Autodesk Inventor part; units mm, degrees
ref_plane "YZ Plane" through (0, 0, 0) normal (1, 0, 0) x (0, 1, 0)
ref_plane "XZ Plane" through (0, 0, 0) normal (0, 1, 0) x (-1, 0, 0)
ref_plane "XY Plane" through (0, 0, 0) normal (0, 0, 1) x (1, 0, 0)
sketch "Sketch1" plane through (0, 0, 0) normal (0, 1, 0) x (-1, 0, 0)
  circle A0 centre (0, 0) radius 1.2
  circle A1 centre (0, 0) radius 3.2
  line L0 (3.2, 0) -> (-3.2, 0) construction
  line L1 (-3.2, 0) -> (-3.2, -15)
  line L2 (-3.2, -15) -> (3.2, -15)
  line L3 (3.2, -15) -> (3.2, 0)
  point P0 (-3.2, 0)
  dimension "d0" = 2.4
  dimension "d1" = 2
  dimension "d2" = 15
extrude "Extrusion1" add sketch "Sketch1" along normal blind 10
properties part number "motor viber"
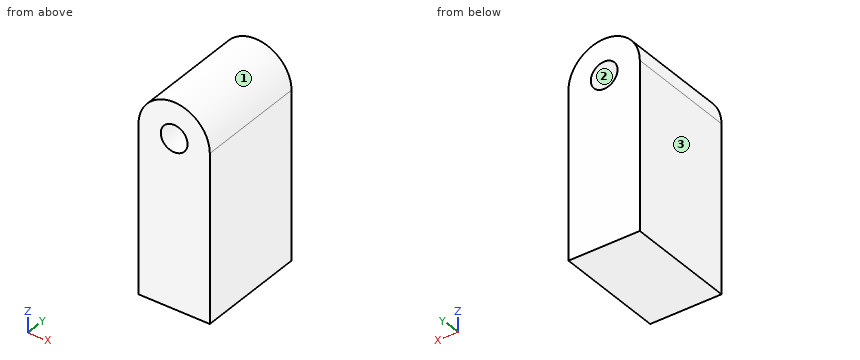
Design review of the part built by this model. Coordinates are the model's own, in mm. Face numbers are marked on the shaded views. Coordinates: 2 decimals unless noted, no trailing zeros. Loops run counter-clockwise (first coordinate to the right, second up) from the corner with the lowest first, then second, coordinate; pieces in that order, holes last. Notation, with made-up numbers: (-22, -19) - (20, -19) arc R16 ccw to (20, -11) - close; hole circle Ø6 at (33.5, -26.5). An arc over 180 degrees is marked (long way). Use CSV: the item, a comma, the result in double quotes. Start each with the question number.
1. Clearance check with a flat-ended pin moving along its axis: pin 1 (2 mm diameter, centred on x = 1, z = -2.5, fed in from -Y). State where the tip first meets the part, or that it passes through.
2. Add section C-C on y = 4. Give the boundary of the cut face in (x, z), plus the area to 3 significant figures.
3. Mouldability with a two-part tool opening along X and no side actions: class the marked faces 1, 2 and 3 as released by +X, released by -X, zero draft, split by the parting line, or undercut.
4. Add section A-A on x = 0. Give the boundary of the cut face in (y, z).
5. To check wall thickness, follow probe 1 along Z at (x, y) = (0, 7.75); probe 2 along X at (y, z) = (7.5, -0.5); probe 3 along Z at (x, y) = (1.25, 7). State the ranges of each line that lie inside material, in increasing order.
6. Add section B-B on z = 0.75. Give the boundary of the cut face in (x, y), plus the area to 3 significant figures.
7. Add section D-D on x = 1.5. Give the boundary of the cut face in (y, z).
Resolved:
1,pin 1,"y = 0"
2,outline,"(-3.2, -15) - (3.2, -15) - (3.2, 0) arc R3.2 ccw to (-3.2, 0) - close; hole circle Ø2.4 at (0, 0)"
2,area,"108 mm2"
3,face 1,"split by the parting line"
3,face 2,"undercut"
3,face 3,"released by -X"
4,outline,"(0, -15) - (10, -15) - (10, -1.2) - (0, -1.2) - close; (0, 1.2) - (10, 1.2) - (10, 3.2) - (0, 3.2) - close"
5,probe 1,"-15 to -1.2, 1.2 to 3.2"
5,probe 2,"-3.2 to -1.09, 1.09 to 3.2"
5,probe 3,"-15 to 2.95"
6,outline,"(-3.11, 0) - (-0.94, 0) - (-0.94, 10) - (-3.11, 10) - close; (0.94, 0) - (3.11, 0) - (3.11, 10) - (0.94, 10) - close"
6,area,"43.5 mm2"
7,outline,"(0, -15) - (10, -15) - (10, 2.83) - (0, 2.83) - close"
